```python
from build123d import *

# Parameters (mm, degrees)
F1_R     = 10.99185
F2_DEPTH = 7


with BuildPart() as f2:
    # F1 (on Top) → F2 (new body)
    with BuildSketch(Plane.XY):
        with BuildLine():
            ThreePointArc((17.033685, 22.367952), (17.930632, 29.765852), (24.81827, 32.610826))
            ThreePointArc((24.81827, 32.610826), (13.218162, 39.29463), (0, 41.419696))
            ThreePointArc((0, 41.419696), (-14.137149, 39.656123), (-27.625239, 35.069115))
            ThreePointArc((-27.625239, 35.069115), (-14.315963, 24.282618), (-10.557758, 7.568515))
            ThreePointArc((-10.557758, 7.568515), (-17.42666, 9.289489), (-24.295563, 7.568515))
            ThreePointArc((-24.295563, 7.568515), (-20.833353, 4.467062), (-19.548337, 0))
            ThreePointArc((-19.548337, 0), (-20.833353, -4.467062), (-24.295563, -7.568515))
            ThreePointArc((-24.295563, -7.568515), (-17.42666, -9.289489), (-10.557758, -7.568515))
            ThreePointArc((-10.557758, -7.568515), (-14.315963, -24.282618), (-27.625239, -35.069115))
            ThreePointArc((-27.625239, -35.069115), (-14.137149, -39.656123), (0, -41.419696))
            ThreePointArc((0, -41.419696), (13.218162, -39.29463), (24.81827, -32.610826))
            ThreePointArc((24.81827, -32.610826), (17.930632, -29.765852), (17.033685, -22.367952))
            ThreePointArc((17.033685, -22.367952), (18.574811, -19.775282), (20.721119, -17.656233))
            ThreePointArc((20.721119, -17.656233), (17.149082, -10.998468), (19.687688, -3.882235))
            ThreePointArc((19.687688, -3.882235), (23.813117, -1.011532), (28.736215, 0))
            ThreePointArc((28.736215, 0), (23.813117, 1.011532), (19.687688, 3.882235))
            ThreePointArc((19.687688, 3.882235), (17.149082, 10.998468), (20.721119, 17.656233))
            ThreePointArc((20.721119, 17.656233), (18.574811, 19.775282), (17.033685, 22.367952))
        make_face()
        with Locations((0, -25.4837)):
            Circle(F1_R, mode=Mode.SUBTRACT)
        Circle(F1_R, mode=Mode.SUBTRACT)
        with Locations((0, 25.4837)):
            Circle(F1_R, mode=Mode.SUBTRACT)
    extrude(amount=F2_DEPTH)


solid = f2.part
```
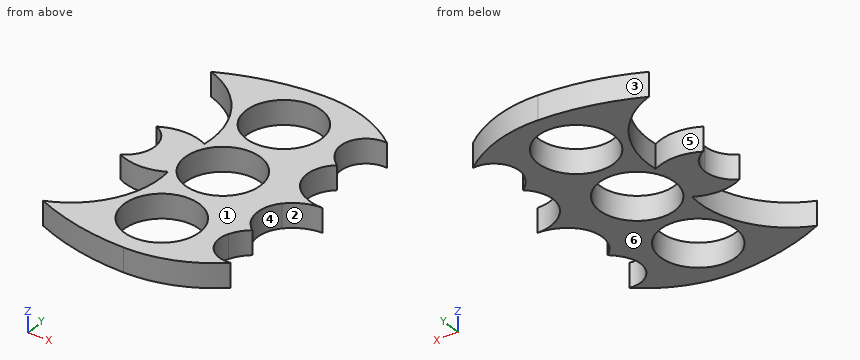
Geometry check sheet. Reference: the model listing, model coordinates, mm. Face numbers are marked on the shaded views. A direction names the side the tool comes from. Coordinates: 2 decimals unless noted, no trailing zeros. Order: outer loops, then holes, each group sorted by start corner. A loop starts at its lowest first (then second) coordinate and runs counter-clockwise, first axis right, second up. Notation, with made-up numbers: M -9,21 L 37,21 A35 ccw 37,58 Z; hole C 67,-3 d5. An arc over 180 degrees is marked long. Answer as a JSON object with one key per item and string values.
Q1. Tool access check on the marked faces 1 and 2. Record the directions out of +Z, -Z, +X, -X, +Y, -Y that give a thin tool (end or side, any length) a straight path to the whole face; none if there is none.
Results are:
{"face 1": "+Z, +X, -X, +Y, -Y", "face 2": "+Z, -Z, +X"}
Q2. Cross-section at C-C on x = -5.5. Record the cut outline in (y, z), and give its area (3 significant figures).
Results are:
{"outline": "M -41.08,0 L -35,0 L -35,7 L -41.08,7 Z; M -15.97,0 L -9.52,0 L -9.52,7 L -15.97,7 Z; M 9.52,0 L 15.97,0 L 15.97,7 L 9.52,7 Z; M 35,0 L 41.08,0 L 41.08,7 L 35,7 Z", "area": "175 mm²"}
Q3. Cross-section at B-B on z = 2.5. Record the cut outline in (x, y).
Results are:
{"outline": "M -27.63,-35.07 A70.06 ccw 0,-41.42 A37.05 ccw 24.82,-32.61 A7.38 cw 17.03,-22.37 A11.84 cw 20.72,-17.66 A9.32 cw 19.69,-3.88 A12.49 cw 28.74,0 A12.49 cw 19.69,3.88 A9.32 cw 20.72,17.66 A11.84 cw 17.03,22.37 A7.38 cw 24.82,32.61 A37.05 ccw 0,41.42 A70.06 ccw -27.63,35.07 A26.11 cw -10.56,7.57 A14.57 ccw -24.3,7.57 A8.41 cw -19.55,0 A8.41 cw -24.3,-7.57 A14.57 ccw -10.56,-7.57 A26.11 cw Z; hole C 0,-25.48 d21.98; hole C 0,0 d21.98; hole C 0,25.48 d21.98"}
Q4. Cross-section at A-A on x = -22.5. Record the cut outline in (y, z), and give its area (3 significant figures).
Results are:
{"outline": "M -37.18,0 L -32.55,0 L -32.55,7 L -37.18,7 Z; M -8.38,0 L -6.4,0 L -6.4,7 L -8.38,7 Z; M 6.4,0 L 8.38,0 L 8.38,7 L 6.4,7 Z; M 32.55,0 L 37.18,0 L 37.18,7 L 32.55,7 Z", "area": "92.5 mm²"}
Q5. Cross-section at D-D on x = 14. Record the cut outline in (y, z), and give its area (3 significant figures).
Results are:
{"outline": "M -39.01,0 L 39.01,0 L 39.01,7 L -39.01,7 Z", "area": "546 mm²"}
Q6. Scan lines: line 1 (Y direction, x = 0, z = 2.5); line 2 (Y direction, x = -13, z = 5.5); line 3 (Y direction, x = -10, z = 3.5). Record each from-to range of solid material in increasing order.
Results are:
{"line 1": "y = -41.42 to -36.48, -14.49 to -10.99, 10.99 to 14.49, 36.48 to 41.42", "line 2": "y = -39.91 to -21.89, -8.6 to 8.6, 21.89 to 39.91", "line 3": "y = -40.48 to -30.05, -20.92 to -4.56, 4.56 to 20.92, 30.05 to 40.48"}
Q7. Depth check by flat-ended pin: pin 1 Ø6 at (x, y) = (-6.5, -28) entering from -Z; pin 2 Ø3 at (y, z) = (-29, 4.5) entering from -X. Enter the tip coordinate at first touch or a pass-through.
Results are:
{"pin 1": "passes through", "pin 2": "stops at x = -19.7"}
Q8. Release check for a two-part mould opening along X. For the marked faces 3, 4, 5 and 6 record: released by +X, released by -X, zero draft, split by the parting line, or undercut.
Results are:
{"face 3": "released by -X", "face 4": "released by +X", "face 5": "undercut", "face 6": "zero draft"}
